The drawing under review shows one solid part. Ordinate dimensions are in mm from its lowest x, y, z. Coordinates: 2 decimals unless noted, no trailing zeros. Order: outer loops, then holes, each group sorted by start corner. A loop starts at its lowest first (then second) coordinate and runs counter-clockwise, first axis right, second up. Notation, with made-up numbers: M 88,77.5 L 108,77.5 A20 ccw 108,86.5 Z; hole C -10,78.5 d7. An arc over 180 degrees is marked long. Answer as a JSON object with one key per item and string values.
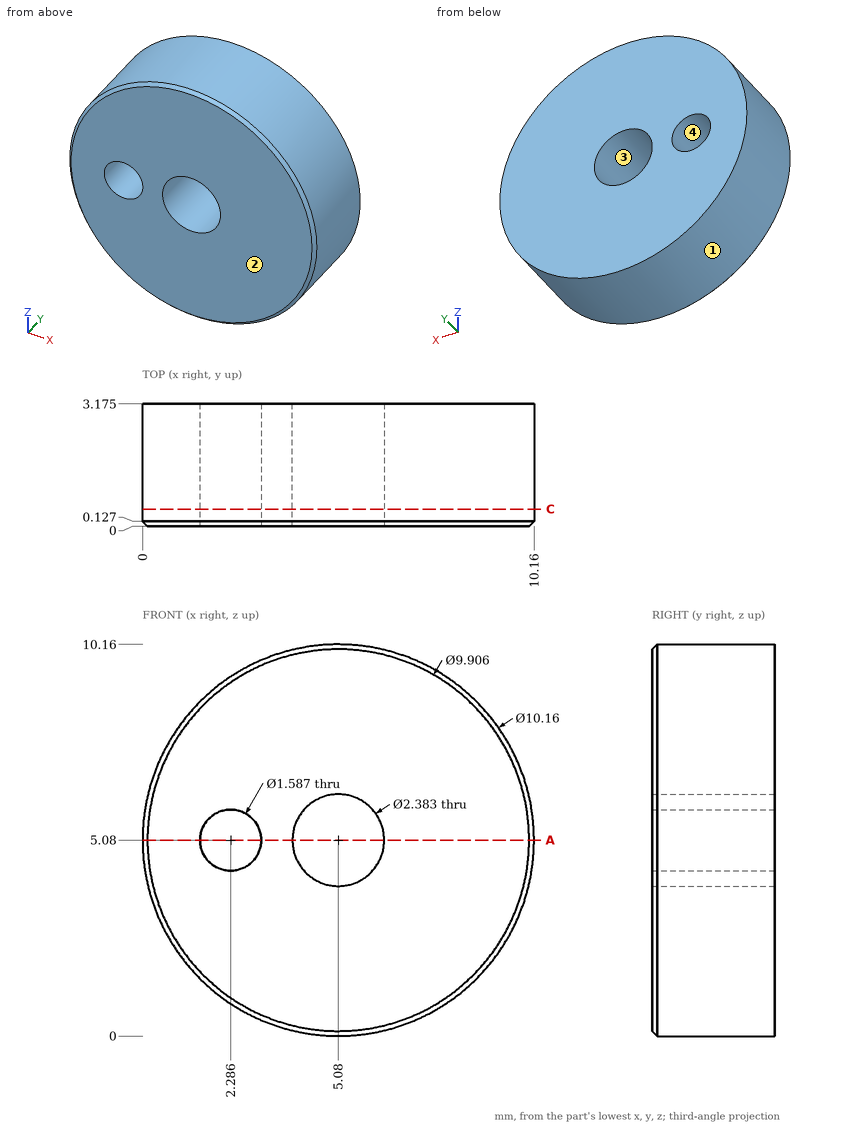
1) Add section C-C (y = 0.45). State the section outline as (x, z) points (1 decimal).
Taken from the geometry:
{"outline": "C 5.1,5.1 d10.2; hole C 2.3,5.1 d1.6; hole C 5.1,5.1 d2.4"}
2) Insertion check: pin 1 Ø1.5 at (y, z) = (1, 8.5) entering from +X. The pin has a flat end and moves straight along its axis. Give the tip position at first contact, or say it passes through.
Taken from the geometry:
{"pin 1": "stops at x = 9.4"}
3) To check wall thickness, follow L1, parallel to Z at x = 5.08, y = 0.8; L2, parallel to X at y = 0.9, z = 5 (1 decimal); L3, parallel to Z at x = 2, y = 1.9. State the ranges of each line that lie inside material, in increasing order.
Taken from the geometry:
{"L1": "z = 0 to 3.89, 6.27 to 10.16", "L2": "x = 0 to 1.5, 3.1 to 3.9, 6.3 to 10.2", "L3": "z = 1.04 to 4.34, 5.82 to 9.12"}
4) Mouldability with a two-part tool opening along Z and no side actions: class the marked faces 1, 2, 3 and 4 as released by +Z, released by -Z, zero draft, split by the parting line, or undercut.
Taken from the geometry:
{"face 1": "split by the parting line", "face 2": "zero draft", "face 3": "undercut", "face 4": "undercut"}
5) Add section A-A (z = 5.08). Count the separate pieces of the cut face and the enclosed holes in it.
Taken from the geometry:
{"separate pieces": "3", "enclosed holes": "0"}
